Autodesk Inventor part; units mm, degrees
ref_plane "YZ Plane" through (0, 0, 0) normal (1, 0, 0) x (0, 1, 0)
ref_plane "XZ Plane" through (0, 0, 0) normal (0, 1, 0) x (-1, 0, 0)
ref_plane "XY Plane" through (0, 0, 0) normal (0, 0, 1) x (1, 0, 0)
sketch "Sketch1" plane through (0, 0, 0) normal (0, 1, 0) x (-1, 0, 0)
  line L0 (0, 0) -> (-9.9, 0)
  line L1 (0, 0) -> (0, -10.3)
  line L2 (0, -10.3) -> (-9.9, -10.3)
  line L3 (-9.9, -10.3) -> (-9.9, 0)
  line L4 (-9.9, -10.3) -> (-9.4, -10.3)
  line L5 (-9.4, -10.3) -> (-9.4, 0)
  line L6 (0, -10.3) -> (-0.5, -10.3)
  line L7 (-0.5, -10.3) -> (-0.5, 0)
  line L8 (-0.5, 0.85) -> (-9.9, 0.85)
  line L9 (-9.9, 0.85) -> (-9.9, 0)
  line L10 (0, 0) -> (0, 0.85)
  line L11 (0, 0.85) -> (-0.5, 0.85)
  line L12 (0, -10.3) -> (0, -11.15)
  line L13 (0, -11.15) -> (-9.9, -11.15)
  line L14 (-9.9, -11.15) -> (-9.9, -10.3)
  line L15 (-9.9, -11.15) -> (-19.8, -11.15)
  line L16 (-19.8, -11.15) -> (-19.8, -10.3)
  line L17 (-19.8, -10.3) -> (-19.8, 0)
  line L18 (-19.3, -10.3) -> (-19.3, 0)
  line L19 (-9.9, -10.3) -> (-19.8, -10.3)
  line L20 (-10.4, -10.3) -> (-10.4, 0)
  line L21 (-9.9, 0) -> (-9.9, -10.3)
  line L22 (-9.9, 0) -> (-9.9, 0.85)
  line L23 (-9.9, 0.85) -> (-10.4, 0.85)
  line L24 (-10.4, 0.85) -> (-19.8, 0.85)
  line L25 (-9.9, 0) -> (-19.8, 0)
  line L26 (-19.8, 0.85) -> (-19.8, 0)
  line L27 (-19.8, -11.15) -> (-29.7, -11.15)
  line L28 (-29.7, -11.15) -> (-29.7, -10.3)
  line L29 (-29.7, -10.3) -> (-29.7, 0)
  line L30 (-29.2, -10.3) -> (-29.2, 0)
  line L31 (-19.8, -10.3) -> (-29.7, -10.3)
  line L32 (-20.3, -10.3) -> (-20.3, 0)
  line L33 (-19.8, 0) -> (-19.8, -10.3)
  line L34 (-19.8, 0) -> (-19.8, 0.85)
  line L35 (-19.8, 0.85) -> (-20.3, 0.85)
  line L36 (-20.3, 0.85) -> (-29.7, 0.85)
  line L37 (-19.8, 0) -> (-29.7, 0)
  line L38 (-29.7, 0.85) -> (-29.7, 0)
  line L39 (-29.7, -11.15) -> (-39.6, -11.15)
  line L40 (-39.6, -11.15) -> (-39.6, -10.3)
  line L41 (-39.6, -10.3) -> (-39.6, 0)
  line L42 (-39.1, -10.3) -> (-39.1, 0)
  line L43 (-29.7, -10.3) -> (-39.6, -10.3)
  line L44 (-30.2, -10.3) -> (-30.2, 0)
  line L45 (-29.7, 0) -> (-29.7, -10.3)
  line L46 (-29.7, 0) -> (-29.7, 0.85)
  line L47 (-29.7, 0.85) -> (-30.2, 0.85)
  line L48 (-30.2, 0.85) -> (-39.6, 0.85)
  line L49 (-29.7, 0) -> (-39.6, 0)
  line L50 (-39.6, 0.85) -> (-39.6, 0)
  line L51 (-39.6, -11.15) -> (-49.5, -11.15)
  line L52 (-49.5, -11.15) -> (-49.5, -10.3)
  line L53 (-49.5, -10.3) -> (-49.5, 0)
  line L54 (-49, -10.3) -> (-49, 0)
  line L55 (-39.6, -10.3) -> (-49.5, -10.3)
  line L56 (-40.1, -10.3) -> (-40.1, 0)
  line L57 (-39.6, 0) -> (-39.6, -10.3)
  line L58 (-39.6, 0) -> (-39.6, 0.85)
  line L59 (-39.6, 0.85) -> (-40.1, 0.85)
  line L60 (-40.1, 0.85) -> (-49.5, 0.85)
  line L61 (-39.6, 0) -> (-49.5, 0)
  line L62 (-49.5, 0.85) -> (-49.5, 0)
  line L63 (-49.5, -11.15) -> (-59.4, -11.15)
  line L64 (-59.4, -11.15) -> (-59.4, -10.3)
  line L65 (-59.4, -10.3) -> (-59.4, 0)
  line L66 (-58.9, -10.3) -> (-58.9, 0)
  line L67 (-49.5, -10.3) -> (-59.4, -10.3)
  line L68 (-50, -10.3) -> (-50, 0)
  line L69 (-49.5, 0) -> (-49.5, -10.3)
  line L70 (-49.5, 0) -> (-49.5, 0.85)
  line L71 (-49.5, 0.85) -> (-50, 0.85)
  line L72 (-50, 0.85) -> (-59.4, 0.85)
  line L73 (-49.5, 0) -> (-59.4, 0)
  line L74 (-59.4, 0.85) -> (-59.4, 0)
  line L75 (-59.4, -11.15) -> (-69.3, -11.15)
  line L76 (-69.3, -11.15) -> (-69.3, -10.3)
  line L77 (-69.3, -10.3) -> (-69.3, 0)
  line L78 (-68.8, -10.3) -> (-68.8, 0)
  line L79 (-59.4, -10.3) -> (-69.3, -10.3)
  line L80 (-59.9, -10.3) -> (-59.9, 0)
  line L81 (-59.4, 0) -> (-59.4, -10.3)
  line L82 (-59.4, 0) -> (-59.4, 0.85)
  line L83 (-59.4, 0.85) -> (-59.9, 0.85)
  line L84 (-59.9, 0.85) -> (-69.3, 0.85)
  line L85 (-59.4, 0) -> (-69.3, 0)
  line L86 (-69.3, 0.85) -> (-69.3, 0)
  line L87 (-69.3, -11.15) -> (-79.2, -11.15)
  line L88 (-79.2, -11.15) -> (-79.2, -10.3)
  line L89 (-79.2, -10.3) -> (-79.2, 0)
  line L90 (-78.7, -10.3) -> (-78.7, 0)
  line L91 (-69.3, -10.3) -> (-79.2, -10.3)
  line L92 (-69.8, -10.3) -> (-69.8, 0)
  line L93 (-69.3, 0) -> (-69.3, -10.3)
  line L94 (-69.3, 0) -> (-69.3, 0.85)
  line L95 (-69.3, 0.85) -> (-69.8, 0.85)
  line L96 (-69.8, 0.85) -> (-79.2, 0.85)
  line L97 (-69.3, 0) -> (-79.2, 0)
  line L98 (-79.2, 0.85) -> (-79.2, 0)
  line L99 (-79.2, -11.15) -> (-89.1, -11.15)
  line L100 (-89.1, -11.15) -> (-89.1, -10.3)
  line L101 (-89.1, -10.3) -> (-89.1, 0)
  line L102 (-88.6, -10.3) -> (-88.6, 0)
  line L103 (-79.2, -10.3) -> (-89.1, -10.3)
  line L104 (-79.7, -10.3) -> (-79.7, 0)
  line L105 (-79.2, 0) -> (-79.2, -10.3)
  line L106 (-79.2, 0) -> (-79.2, 0.85)
  line L107 (-79.2, 0.85) -> (-79.7, 0.85)
  line L108 (-79.7, 0.85) -> (-89.1, 0.85)
  line L109 (-79.2, 0) -> (-89.1, 0)
  line L110 (-89.1, 0.85) -> (-89.1, 0)
  line L111 (-89.1, -11.15) -> (-99, -11.15)
  line L112 (-99, -11.15) -> (-99, -10.3)
  line L113 (-99, -10.3) -> (-99, 0)
  line L114 (-98.5, -10.3) -> (-98.5, 0)
  line L115 (-89.1, -10.3) -> (-99, -10.3)
  line L116 (-89.6, -10.3) -> (-89.6, 0)
  line L117 (-89.1, 0) -> (-89.1, -10.3)
  line L118 (-89.1, 0) -> (-89.1, 0.85)
  line L119 (-89.1, 0.85) -> (-89.6, 0.85)
  line L120 (-89.6, 0.85) -> (-99, 0.85)
  line L121 (-89.1, 0) -> (-99, 0)
  line L122 (-99, 0.85) -> (-99, 0)
  line L123 (0, -11.15) -> (0, 0.85)
  line L124 (0, -11.15) -> (0, -12.65)
  line L125 (0, -12.65) -> (1.5, -12.65)
  line L126 (-99, 0.85) -> (-100.5, 0.85)
  line L127 (-100.5, 0.85) -> (-100.5, 2.35)
  line L128 (1.5, -12.65) -> (-100.5, -12.65)
  line L129 (-100.5, -12.65) -> (-100.5, 2.35)
  line L130 (-100.5, 2.35) -> (1.5, 2.35)
  line L131 (1.5, 2.35) -> (1.5, -12.65)
  line L132 (0, -11.15) -> (1.5, -11.15)
  line L133 (0, 0.85) -> (1.5, 0.85)
  line L134 (0, -11.15) -> (-2, -11.15)
  line L135 (-2, -11.15) -> (-2, 0.85)
  line L136 (-0.5, -10.3) -> (-1.5, -10.3)
  line L137 (-1.5, -10.3) -> (-0.5, -9.3)
  line L138 (-9.4, -10.3) -> (-8.4, -10.3)
  line L139 (-8.4, -10.3) -> (-9.4, -9.3)
  line L140 (-9.4, 0) -> (-9.4, -1)
  line L141 (-9.4, -1) -> (-8.4, 0)
  line L142 (-2, 0) -> (-3, 0)
  line L143 (-0.5, 0) -> (-1.5, 0)
  line L144 (-1.5, 0) -> (-0.5, -1)
  dimension "d0" = 9.9
  dimension "d1" = 10.3
  dimension "d2" = 0.5
  dimension "d3" = 0.5
  dimension "d6" = 0.85
  dimension "d7" = 0.85
  dimension "d10" = 9.9
  dimension "d15" = 1.5
  dimension "d16" = 1.5
  dimension "d19" = 1.5
  dimension "d20" = 2
  dimension "d26" = 1
  dimension "d27" = 45
  dimension "d28" = 1
  dimension "d29" = 1
  dimension "d30" = 1
  dimension "d31" = 1
extrude "Extrusion1" add sketch "Sketch1" along normal blind 6 contours L1 L2 L7 L0 | L0 L135 L8 L11 L10 | L12 L13 L135 L2 | L0 L9 L8 L135 | L13 L14 L2 L135 | L3 L0 L5 L2
extrude "Extrusion2" add sketch "Sketch1" along normal blind 5 contours L7 L144 L0 | L2 L137 L7 | L141 L5 L0 | L2 L5 L139
pattern_linear "Rectangular Pattern1" count 4 spacing 9.9 along (1, 0, 0) of "Extrusion1", "Extrusion2"
equation "\"d25\" = d10"
properties part number "4x led strip divider"
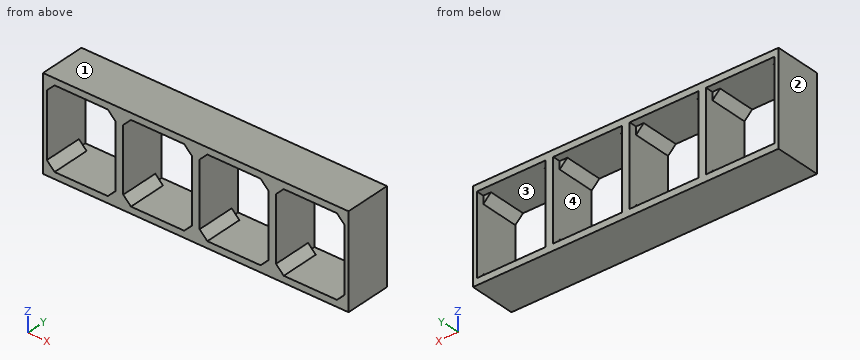
Input: part model. Units: mm. Frame: model coordinates. Face numbers are marked on the shaded views. Give positions to 0.01 mm unless a question says otherwise; leave off trailing zeros. Write each loop counter-clockwise with the first axis right and the second up, starting at its lowest first coordinate (ties: lowest second). Pieces come first, ordered by that corner, then holes.
Q1. Material intervals for probe 1 along X at (y, z) = (3, -6); probe 2 along Z at (x, y) = (32, 0.4); probe 3 along Z at (x, y) = (18.5, 0.5), sorted ascending.
Q2. Pull-direction query (X, two-part tool) for the marked faces 1, 2, 3 and 4; classes: pulls with the +X half, pulls with the -X half, needs draft (parallel to the pull), parting line crosses it, or undercut.
Q3. Section B-B, the plane z = -8.25. Output: boundary loops of the cut face in (x, y).
Q4. Section C-C, the plane y = 1.55. State how many separate pieces and enclosed holes the cut face has, plus the area to 3 significant figures.
Q5. Section A-A, the plane x = 27. Output: boundary loops of the cut face in (y, z), plus the area to 3 significant figures.
Q6. First-contact query: P1, Ø3, axis at x = 5.5, z = -2.5, coming from the -Y side; P2, Ø0.5, axis at x = 1, z = -9.5, coming from the +Y side. Flat tips, straight axial feed; report the tip coordinate or a pass-through.
Filled in:
1. probe 1: x = 0 to 0.5, 9.4 to 10.4, 19.3 to 20.3, 29.2 to 30.2, 39.1 to 39.6
1. probe 2: z = -11.15 to -10.3, 0 to 0.85
1. probe 3: z = -11.15 to -10.1, -0.2 to 0.85
2. face 1: needs draft
2. face 2: pulls with the -X half
2. face 3: undercut
2. face 4: undercut
3. outline: (0, 0) - (0.5, 0) - (0.5, 6) - (0, 6) - close; (9.4, 0) - (10.4, 0) - (10.4, 6) - (9.4, 6) - close; (19.3, 0) - (20.3, 0) - (20.3, 6) - (19.3, 6) - close; (29.2, 0) - (30.2, 0) - (30.2, 6) - (29.2, 6) - close; (39.1, 0) - (39.6, 0) - (39.6, 6) - (39.1, 6) - close
4. separate pieces: 1
4. enclosed holes: 4
4. area: 117 mm2
5. outline: (0, -11.15) - (6, -11.15) - (6, -10.3) - (0, -10.3) - close; (0, 0) - (6, 0) - (6, 0.85) - (0, 0.85) - close
5. area: 10.2 mm2
6. P1: passes through
6. P2: stops at y = 5
